Check sheet for the modelled part. Datum: model origin and axes. Units: mm. A direction names the side the tool comes from. Coordinates: 2 decimals unless noted, no trailing zeros. Order: outer loops, then holes, each group sorted by start corner. A loop starts at its lowest first (then second) coordinate and runs counter-clockwise, first axis right, second up.
from build123d import *

# Parameters (mm, degrees)
F0_W      = 76.2
F0_H      = 76.2
F1_DEPTH  = 76.2
F2_R      = 19.9669900024
F3_DEPTH  = 12.7
F5_DEPTH  = 12.7
F6_W      = 38.1
F6_H      = 38.1
F7_DEPTH  = 12.7
F9_DEPTH  = 12.7
F11_DEPTH = 12.7
F13_DEPTH = 12.7


with BuildPart() as f1:
    # F0 (on Front) → F1 (new body)
    with BuildSketch(Plane.XZ):
        Rectangle(F0_W, F0_H)
    extrude(amount=F1_DEPTH)

    # F2 (on face) → F3 (cut)
    with BuildSketch(Plane.XZ.offset(76.2)):
        Circle(F2_R)
    extrude(amount=-F3_DEPTH, mode=Mode.SUBTRACT)

    # F4 (on face) → F5 (cut)
    with BuildSketch(Plane.XY.offset(38.1)):
        Polygon((17.6528156414, -48.2918578625), (0, -17.716284275), (-17.6528156414, -48.2918578625), align=None)
    extrude(amount=-F5_DEPTH, mode=Mode.SUBTRACT)

    # F6 (on face) → F7 (cut)
    with BuildSketch(Plane.YZ.offset(38.1)):
        with Locations((-38.1, 0)):
            Rectangle(F6_W, F6_H)
    extrude(amount=-F7_DEPTH, mode=Mode.SUBTRACT)

    # F8 (on face) → F9 (cut)
    with BuildSketch(Plane(origin=(-38.1, 0, 0), x_dir=(0, -1, 0), z_dir=(-1, 0, 0))):
        Polygon((38.1, -11.9736748281), (50.0736748281, -23.9473496562), (62.0473496562, -11.9736748281), (50.0736748281, 0), (62.0473496562, 11.9736748281), (50.0736748281, 23.9473496562), (38.1, 11.9736748281), (26.1263251719, 23.9473496562), (14.1526503438, 11.9736748281), (26.1263251719, 0), (14.1526503438, -11.9736748281), (26.1263251719, -23.9473496562), align=None)
    extrude(amount=-F9_DEPTH, mode=Mode.SUBTRACT)

    # F10 (on face) → F11 (cut)
    with BuildSketch(Plane(origin=(0, 0, 0), x_dir=(-1, 0, 0), z_dir=(0, 1, 0))):
        Polygon((-12.7, 21.9970452561), (-25.4, 0), (-12.7, -21.9970452561), (12.7, -21.9970452561), (25.4, 0), (12.7, 21.9970452561), align=None)
    extrude(amount=-F11_DEPTH, mode=Mode.SUBTRACT)

    # F12 (on face) → F13 (cut)
    with BuildSketch(Plane(origin=(0, 0, -38.1), x_dir=(1, 0, 0), z_dir=(0, 0, -1))):
        Polygon((-9.2270901057, 44.0961266285), (2.1782204995, 47.8019366858), (-9.2270901057, 63.5), align=None)
        Polygon((-9.2270901057, 32.1038733715), (-9.2270901057, 44.0961266285), (-27.681270317, 38.1), align=None)
        Polygon((9.2270901057, 38.1), (2.1782204995, 47.8019366858), (-9.2270901057, 44.0961266285), (-9.2270901057, 32.1038733715), (2.1782204995, 28.3980633142), align=None)
        Polygon((-9.2270901057, 12.7), (2.1782204995, 28.3980633142), (-9.2270901057, 32.1038733715), align=None)
        Polygon((20.6324007108, 22.4019366858), (9.2270901057, 38.1), (2.1782204995, 28.3980633142), align=None)
        Polygon((9.2270901057, 38.1), (20.6324007108, 53.7980633142), (2.1782204995, 47.8019366858), align=None)
    extrude(amount=-F13_DEPTH, mode=Mode.SUBTRACT)


solid = f1.part
(1) Cross-section at D-D (x = -15). Enter the section's corners in (y, z), and give its area (3 significant figures).
Filled in:
outline: (-76.2, -38.1) - (-42.22, -38.1) - (-42.22, -25.4) - (-33.98, -25.4) - (-33.98, -38.1) - (0, -38.1) - (0, -18.01) - (-12.7, -18.01) - (-12.7, 18.01) - (0, 18.01) - (0, 38.1) - (-43.7, 38.1) - (-43.7, 25.4) - (-48.29, 25.4) - (-48.29, 38.1) - (-76.2, 38.1) - (-76.2, 13.18) - (-63.5, 13.18) - (-63.5, -13.18) - (-76.2, -13.18) - close
area: 4,850 mm2
(2) Release check for a two-part mould opening along Y. For faces 1 (the flat face through (0, -6, 21.997)), 2 (the flat face through (16, -76.2, 17)), 3 (the flat face through (14.85, -45.84, -31.84)) record: +Y half, -Y half, draft (parallel to the pull), parting line (faces both ways), or undercut.
Filled in:
face 1: draft
face 2: -Y half
face 3: undercut
(3) Thickness scan on probe 1 along Y at (x, z) = (26, -3); probe 2 along Z at (x, y) = (0, -67); probe 3 along Z at (x, y) = (-26, -59.5). Record the ranges inside material, lowest first.
Filled in:
probe 1: y = -76.2 to -57.15, -19.05 to 0
probe 2: z = -38.1 to -19.97, 19.97 to 38.1
probe 3: z = -38.1 to -14.52, -9.43 to 9.43, 14.52 to 38.1
(4) Cross-section at B-B (x = -31.5). Enter the section's corners in (y, z), and give its area (3 significant figures).
Filled in:
outline: (-76.2, -38.1) - (0, -38.1) - (0, 38.1) - (-76.2, 38.1) - close; hole (-62.05, -11.97) - (-50.07, -23.95) - (-38.1, -11.97) - (-26.13, -23.95) - (-14.15, -11.97) - (-26.13, 0) - (-14.15, 11.97) - (-26.13, 23.95) - (-38.1, 11.97) - (-50.07, 23.95) - (-62.05, 11.97) - (-50.07, 0) - close
area: 4,370 mm2
(5) Go/stop test with flat-tipped pins: P1, Ø24, axis at x = 6, y = -45.5, coming from the -Z side; P2, Ø13, axis at x = 5.5, z = 0.5, coming from the +Y side; P3, Ø10, axis at y = -47, z = 8, coming from the -X side; P4, Ø12, axis at x = -8, z = 9.5, coming from the -Y side. Record where each tip stops, or that it passes through.
Filled in:
P1: stops at z = -38.1
P2: stops at y = -12.7
P3: stops at x = -25.4
P4: stops at y = -63.5
(6) Cross-section at C-C (y = -52). Enter the section's corners in (x, z), and give its area (3 significant figures).
Filled in:
outline: (-38.1, -38.1) - (-9.23, -38.1) - (-9.23, -25.4) - (-0.87, -25.4) - (-0.87, -38.1) - (15.1, -38.1) - (15.1, -25.4) - (19.33, -25.4) - (19.33, -38.1) - (38.1, -38.1) - (38.1, -19.05) - (25.4, -19.05) - (25.4, 19.05) - (38.1, 19.05) - (38.1, 38.1) - (-38.1, 38.1) - (-38.1, 22.02) - (-25.4, 22.02) - (-25.4, 1.93) - (-38.1, 1.93) - (-38.1, -1.93) - (-25.4, -1.93) - (-25.4, -22.02) - (-38.1, -22.02) - close
area: 4,650 mm2
(7) Cross-section at A-A (y = -9). Enter the section's corners in (x, z), and give its area (3 significant figures).
Filled in:
outline: (-38.1, -38.1) - (38.1, -38.1) - (38.1, 38.1) - (-38.1, 38.1) - close; hole (-25.4, 0) - (-12.7, -22) - (12.7, -22) - (25.4, 0) - (12.7, 22) - (-12.7, 22) - close
area: 4,130 mm2
(8) Tool access check on faces 4 (the flat face through (0, -36, 25.4)), 5 (the flat face through (-9.227, -54, -32)), 6 (the flat face through (-31.84, -20.22, 18.04)). Record the directions out of +Z, -Z, +X, -X, +Y, -Y that give a thin tool (end or side, any length) a straight path to the whole face; none if there is none.
Filled in:
face 4: +Z
face 5: -Z
face 6: -X
